Answer from the drawing. Dimensions are ordinates in mm from the lowest x, y and z of the part. A direction names the side the tool comes from. Coordinates: 2 decimals unless noted, no trailing zeros. Order: outer loops, then holes, each group sorted by start corner. A loop starts at its lowest first (then second) coordinate and runs counter-clockwise, first axis right, second up. Notation, with made-up numbers: M 71.5,28 L 92.5,28 A10 ccw 92.5,38 Z; hole C 19,-5.5 d11. An arc over 180 degrees is marked long. One line per question, with ' | ' between items. Start each with the question number.
1) The mould has two halves that part along X. Classify the marked faces 1, 2, 3 and 4: +X half, -X half, draft (parallel to the pull), parting line (faces both ways), or undercut.
2) Find section D-D, the plane z = 5. Write down the section's boundary in (x, y), plus the area to 3 significant figures.
3) Find section C-C, the plane x = 2.5. Write down the section's boundary in (y, z), plus the area to 3 significant figures.
4) Find section A-A, the plane z = 35. Write down the section's boundary in (x, y).
5) Consider probe 1 along X at (y, z) = (2, 5); probe 2 along Y at (x, z) = (2.5, 30.5); probe 3 along X at (y, z) = (7.75, 28.5). Determine where each line is inside the solid, lowest interval first.
6) Given P1, Ø2, axis at x = 2.5, y = 4.5, coming from the +Z side; P2, Ø8, axis at x = 41, y = 11.5, coming from the +Z side; P3, Ø9.5, axis at x = 26, z = 4, coming from the +Y side; P4, Ø2.5, axis at x = 7, z = 5, coming from the +Y side, each flat-ended and moving along its own axis, determine where each tip first touches the part or whether it passes through.
7) A tool of negligible diameter and unlimited length cuts with its end or side. For the marked faces 5, 6 and 7, from which of +Z, -Z, +X, -X, +Y, -Y can it reach the whole face along a straight path? Write none if from no direction.
8) Find section B-B, the plane y = 12.25. Write down the section's boundary in (x, z), plus the area to 3 significant figures.
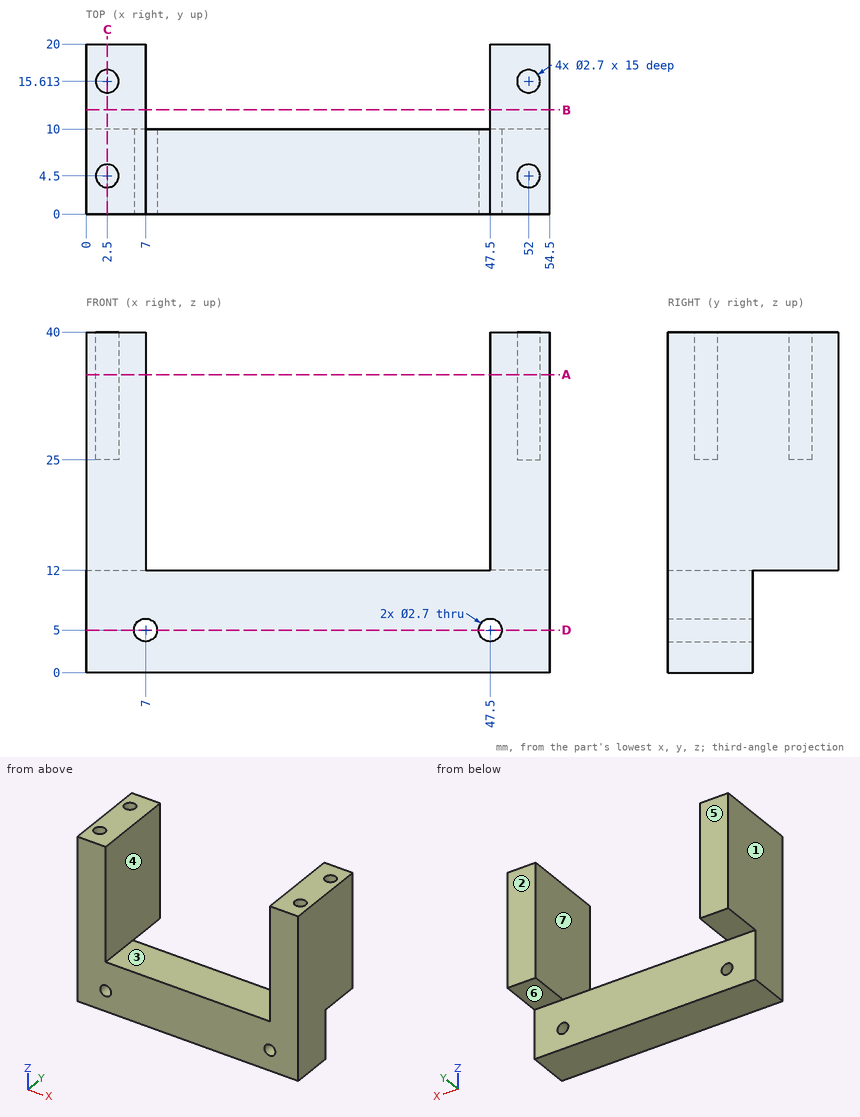
Report:
1) face 1: -X half | face 2: draft | face 3: undercut | face 4: undercut
2) outline: M 0,0 L 5.65,0 L 5.65,10 L 0,10 Z; M 8.35,0 L 46.15,0 L 46.15,10 L 8.35,10 Z; M 48.85,0 L 54.5,0 L 54.5,10 L 48.85,10 Z | area: 491 mm^2
3) outline: M 0,0 L 10,0 L 10,12 L 20,12 L 20,40 L 16.96,40 L 16.96,25 L 14.26,25 L 14.26,40 L 5.85,40 L 5.85,25 L 3.15,25 L 3.15,40 L 0,40 Z | area: 599 mm^2
4) outline: M 0,0 L 7,0 L 7,20 L 0,20 Z; M 47.5,0 L 54.5,0 L 54.5,20 L 47.5,20 Z; hole C 2.5,4.5 d2.7; hole C 2.5,15.61 d2.7; hole C 52,4.5 d2.7; hole C 52,15.61 d2.7
5) probe 1: x = 0 to 5.65, 8.35 to 46.15, 48.85 to 54.5 | probe 2: y = 0 to 3.15, 5.85 to 14.26, 16.96 to 20 | probe 3: x = 0 to 7, 47.5 to 54.5
6) P1: stops at z = 25 | P2: stops at z = 12 | P3: stops at y = 10 | P4: passes through
7) face 5: +Z, -Z, +X, -X, +Y | face 6: -Z, +X, -X, +Y | face 7: +Z, +Y, -Y
8) outline: M 0,12 L 7,12 L 7,40 L 0,40 Z; M 47.5,12 L 54.5,12 L 54.5,40 L 47.5,40 Z | area: 392 mm^2
